from build123d import *

# Parameters (mm, degrees)
SKETCH1_W                   = 116.84
SKETCH1_H                   = 137.16
SKETCH1_R                   = 3.110430672
BOSS_EXTRUDE1_DEPTH         = 5
SKETCH12_W                  = 85
SKETCH12_H                  = 23.975046692
BOSS_EXTRUDE15_DEPTH        = 5
SKETCH17_W                  = 50
SKETCH17_H                  = 50
BOSS_EXTRUDE18_DEPTH        = 6
SKETCH10_W                  = 43
SKETCH10_H                  = 43
BOSS_EXTRUDE19_DEPTH        = 25
SKETCH19_W                  = 55
SKETCH19_H                  = 55
BOSS_EXTRUDE20_DEPTH        = 11
SKETCH20_R                  = 2.25
BOSS_EXTRUDE22_DEPTH        = 25
BOSS_EXTRUDE22_2_DEPTH      = 25
BOSS_EXTRUDE22_3_DEPTH      = 25
BOSS_EXTRUDE22_4_DEPTH      = 25
SKETCH21_W                  = 24.5
SKETCH21_H                  = 21.5
BOSS_EXTRUDE23_DEPTH        = 4
SKETCH21_W_2                = 21.5
SKETCH21_H_2                = 24.5
BOSS_EXTRUDE23_2_DEPTH      = 4
BOSS_EXTRUDE23_3_DEPTH      = 4
BOSS_EXTRUDE23_4_DEPTH      = 4
SKETCH25_R                  = 4
BOSS_EXTRUDE24_DEPTH        = 10
BOSS_EXTRUDE24_DEPTH_BACK   = 3.25
BOSS_EXTRUDE24_2_DEPTH      = 10
BOSS_EXTRUDE24_2_DEPTH_BACK = 3.25
BOSS_EXTRUDE24_3_DEPTH      = 10
BOSS_EXTRUDE24_3_DEPTH_BACK = 3.25
BOSS_EXTRUDE24_4_DEPTH      = 10
BOSS_EXTRUDE24_4_DEPTH_BACK = 3.25


with BuildPart() as part:
    # Sketch1 → Boss-Extrude1 (new body)
    with BuildSketch(Plane(origin=(0, 0, 0), x_dir=(1, 0, 0), z_dir=(0, 1, 0))):
        with Locations((-0.693486938, -16.384561015)):
            Rectangle(SKETCH1_W, SKETCH1_H)
        with Locations((-51.493486938, 44.575438985)):
            Circle(SKETCH1_R, mode=Mode.SUBTRACT)
        with Locations((50.106513062, -57.024561015)):
            Circle(SKETCH1_R, mode=Mode.SUBTRACT)
        with Locations((-51.493486938, -57.024561015)):
            Circle(SKETCH1_R, mode=Mode.SUBTRACT)
        with Locations((50.106513062, 44.575438985)):
            Circle(SKETCH1_R, mode=Mode.SUBTRACT)
    extrude(amount=-BOSS_EXTRUDE1_DEPTH)


with BuildPart() as body_2:
    # Sketch12 → Boss-Extrude15 (new body)
    with BuildSketch(Plane(origin=(0, 0, 0), x_dir=(1, 0, 0), z_dir=(0, 1, 0))):
        with Locations((0, 58)):
            Rectangle(SKETCH12_W, SKETCH12_H)
    extrude(amount=BOSS_EXTRUDE15_DEPTH)


with BuildPart() as body_3:
    # Sketch17 → Boss-Extrude18 (new body)
    with BuildSketch(Plane(origin=(0, 0, 0), x_dir=(1, 0, 0), z_dir=(0, 1, 0))):
        with Locations((-0.7, -7.31)):
            Rectangle(SKETCH17_W, SKETCH17_H)
    extrude(amount=-BOSS_EXTRUDE18_DEPTH)


with BuildPart() as body_4:
    # Sketch10 → Boss-Extrude19 (new body, symmetric)
    with BuildSketch(Plane(origin=(0, 0, 0), x_dir=(1, 0, 0), z_dir=(0, 1, 0))):
        with Locations((-0.695517903, -7.307291257)):
            Rectangle(SKETCH10_W, SKETCH10_H)
    extrude(amount=BOSS_EXTRUDE19_DEPTH, both=True)


with BuildPart() as body_5:
    # Sketch19 → Boss-Extrude20 (new body)
    with BuildSketch(Plane(origin=(0, 0, 0), x_dir=(1, 0, 0), z_dir=(0, 1, 0))):
        with Locations((-0.7, -7.31)):
            Rectangle(SKETCH19_W, SKETCH19_H)
    extrude(amount=-BOSS_EXTRUDE20_DEPTH)


with BuildPart() as part_1:
    add(part.part)

    # Combine1: cut body 2
    add(body_2.part, mode=Mode.SUBTRACT)


with BuildPart() as body_3_1:
    # Body-Move/Copy4: moved
    add(body_3.part.moved(Location((0, -6, 0))))


with BuildPart() as body_5_1:
    add(body_5.part)

    # Combine4: cut body 3
    add(body_3_1.part, mode=Mode.SUBTRACT)

    # Combine7: union part
    add(part_1.part)

    # Combine8: cut body 4
    add(body_4.part, mode=Mode.SUBTRACT)


with BuildPart() as body_2_2:
    # Sketch20 → Boss-Extrude22 (new body, symmetric)
    with BuildSketch(Plane(origin=(0, 0, 0), x_dir=(1, 0, 0), z_dir=(0, 1, 0))):
        with Locations((33.02, 33.02)):
            Circle(SKETCH20_R)
    extrude(amount=BOSS_EXTRUDE22_DEPTH, both=True)


with BuildPart() as body_3_2:
    # Sketch20 → Boss-Extrude22 2 (new body, symmetric)
    with BuildSketch(Plane(origin=(0, 0, 0), x_dir=(1, 0, 0), z_dir=(0, 1, 0))):
        with Locations((33.02, -33.02)):
            Circle(SKETCH20_R)
    extrude(amount=BOSS_EXTRUDE22_2_DEPTH, both=True)


with BuildPart() as body_4_2:
    # Sketch20 → Boss-Extrude22 3 (new body, symmetric)
    with BuildSketch(Plane(origin=(0, 0, 0), x_dir=(1, 0, 0), z_dir=(0, 1, 0))):
        with Locations((-33.02, -33.02)):
            Circle(SKETCH20_R)
    extrude(amount=BOSS_EXTRUDE22_3_DEPTH, both=True)


with BuildPart() as body_5_2:
    # Sketch20 → Boss-Extrude22 4 (new body, symmetric)
    with BuildSketch(Plane(origin=(0, 0, 0), x_dir=(1, 0, 0), z_dir=(0, 1, 0))):
        with Locations((-33.02, 33.02)):
            Circle(SKETCH20_R)
    extrude(amount=BOSS_EXTRUDE22_4_DEPTH, both=True)


with BuildPart() as body_5_3:
    add(body_5_1.part)

    # Combine9: cut body 4 2, body 3 2, body 2 2, body 5 2
    add(body_4_2.part, mode=Mode.SUBTRACT)
    add(body_3_2.part, mode=Mode.SUBTRACT)
    add(body_2_2.part, mode=Mode.SUBTRACT)
    add(body_5_2.part, mode=Mode.SUBTRACT)


with BuildPart() as body_2_3:
    # Sketch21 → Boss-Extrude23 (new body)
    with BuildSketch(Plane(origin=(0, 0, 0), x_dir=(1, 0, 0), z_dir=(0, 1, 0))):
        with Locations((-0.69, 27.145438985)):
            Rectangle(SKETCH21_W, SKETCH21_H)
    extrude(amount=-BOSS_EXTRUDE23_DEPTH)


with BuildPart() as body_3_3:
    # Sketch21 → Boss-Extrude23 2 (new body)
    with BuildSketch(Plane(origin=(0, 0, 0), x_dir=(1, 0, 0), z_dir=(0, 1, 0))):
        with Locations((32.676513062, -6.25)):
            Rectangle(SKETCH21_W_2, SKETCH21_H_2)
    extrude(amount=-BOSS_EXTRUDE23_2_DEPTH)


with BuildPart() as body_4_3:
    # Sketch21 → Boss-Extrude23 3 (new body)
    with BuildSketch(Plane(origin=(0, 0, 0), x_dir=(1, 0, 0), z_dir=(0, 1, 0))):
        with Locations((-34.063486938, -6.25)):
            Rectangle(SKETCH21_W_2, SKETCH21_H_2)
    extrude(amount=-BOSS_EXTRUDE23_3_DEPTH)


with BuildPart() as body_5_3_1:
    # Sketch21 → Boss-Extrude23 4 (new body)
    with BuildSketch(Plane(origin=(0, 0, 0), x_dir=(1, 0, 0), z_dir=(0, 1, 0))):
        with Locations((-0.69, -39.614561015)):
            Rectangle(SKETCH21_W, SKETCH21_H)
    extrude(amount=-BOSS_EXTRUDE23_4_DEPTH)


with BuildPart() as body_5_4:
    add(body_5_3.part)

    # Combine10: cut body 3 3, body 2 3, body 5 3, body 4 3
    add(body_3_3.part, mode=Mode.SUBTRACT)
    add(body_2_3.part, mode=Mode.SUBTRACT)
    add(body_5_3_1.part, mode=Mode.SUBTRACT)
    add(body_4_3.part, mode=Mode.SUBTRACT)


with BuildPart() as body_2_4:
    # Sketch25 → Boss-Extrude24 (new body, two sides)
    with BuildSketch(Plane(origin=(0, 0, 0), x_dir=(1, 0, 0), z_dir=(0, 1, 0))) as boss_extrude24_sk:
        with Locations((33.02, 33.02)):
            Circle(SKETCH25_R)
    extrude(amount=BOSS_EXTRUDE24_DEPTH)
    extrude(boss_extrude24_sk.sketch, amount=-BOSS_EXTRUDE24_DEPTH_BACK)


with BuildPart() as body_3_4:
    # Sketch25 → Boss-Extrude24 2 (new body, two sides)
    with BuildSketch(Plane(origin=(0, 0, 0), x_dir=(1, 0, 0), z_dir=(0, 1, 0))) as boss_extrude24_2_sk:
        with Locations((-33.02, 33.02)):
            Circle(SKETCH25_R)
    extrude(amount=BOSS_EXTRUDE24_2_DEPTH)
    extrude(boss_extrude24_2_sk.sketch, amount=-BOSS_EXTRUDE24_2_DEPTH_BACK)


with BuildPart() as body_4_4:
    # Sketch25 → Boss-Extrude24 3 (new body, two sides)
    with BuildSketch(Plane(origin=(0, 0, 0), x_dir=(1, 0, 0), z_dir=(0, 1, 0))) as boss_extrude24_3_sk:
        with Locations((-33.02, -33.02)):
            Circle(SKETCH25_R)
    extrude(amount=BOSS_EXTRUDE24_3_DEPTH)
    extrude(boss_extrude24_3_sk.sketch, amount=-BOSS_EXTRUDE24_3_DEPTH_BACK)


with BuildPart() as body_5_4_1:
    # Sketch25 → Boss-Extrude24 4 (new body, two sides)
    with BuildSketch(Plane(origin=(0, 0, 0), x_dir=(1, 0, 0), z_dir=(0, 1, 0))) as boss_extrude24_4_sk:
        with Locations((33.02, -33.02)):
            Circle(SKETCH25_R)
    extrude(amount=BOSS_EXTRUDE24_4_DEPTH)
    extrude(boss_extrude24_4_sk.sketch, amount=-BOSS_EXTRUDE24_4_DEPTH_BACK)


with BuildPart() as body_5_5:
    add(body_5_4.part)

    # Combine11: cut body 4 4, body 3 4, body 2 4, body 5 4
    add(body_4_4.part, mode=Mode.SUBTRACT)
    add(body_3_4.part, mode=Mode.SUBTRACT)
    add(body_2_4.part, mode=Mode.SUBTRACT)
    add(body_5_4_1.part, mode=Mode.SUBTRACT)


solid = body_5_5.part
CAD build for the part. Positions are in the model's coordinates, mm. A direction names the side the tool comes from. Coordinates: 2 decimals unless noted, no trailing zeros. Loops run counter-clockwise (first coordinate to the right, second up) from the corner with the lowest first, then second, coordinate; pieces in that order, holes last. Notation, with made-up numbers: (-33, 87.25) - (1, 87.25) arc R32 cw to (1, 113.25) - close; hole circle Ø10 at (36.5, 59). An arc over 180 degrees is marked (long way). Write item = value, one per line. Start each with the question number.
Q1. Drill centre lines: L1, parallel to Z at x = -33.02, y = -1.35; L2, parallel to Z at x = -33.02, y = -4.4; L3, parallel to X at y = -3.75, z = 33.02. Where is each one in solid material? Low to high.
Q2. Cut at B-B, the plane z = 20.5. List the corners of the cut face in (x, y), then the cut area to 3 significant figures.
Q3. Flat gauge pins, fed straight in: pin 1 Ø10 at (x, z) = (-47, 7) entering from +Y; pin 2 Ø5 at (x, z) = (33.02, 33.02) entering from -Y; pin 3 Ø2.5 at (x, y) = (-7.5, -9.5) entering from +Z; pin 4 Ø2 at (x, y) = (-34, -7.5) entering from -Z. Where does each tip first touch, or does it go through?
Q4. Pull direction Z, two halves, no side cores. Call faces 1 (the flat face through (-12.94, -2, -27)), 2 (the flat face through (-1, -8, -20.19)), 3 (the flat face through (57.727, -2, 17)): pulls with the +Z half, pulls with the -Z half, needs draft (parallel to the pull), parting line crosses it, or undercut.
Q5. Cut at D-D, the plane z = -33.02. List the corners of the cut face in (x, y), then the cut area to 3 significant figures.
Q6. Cut at C-C, the plane x = 33.02. List the corners of the cut face in (y, z), then the cut area to 3 significant figures.
Q7. Cut at A-A, the plane x = 8. List the corners of the cut face in (y, z), then the cut area to 3 significant figures.
Q8. Which spindle directions (+Z, -Z, +X, -X, +Y, -Y) get a long thin tool onto all of the face, cutting with end or side? Do faces 4 (the flat face through (-31, -3.25, -31)), 5 (the flat face through (-1, -4.3, 28.807)), 6 (the flat face through (-2, -2, 84.965)), 7 (the flat face through (-1, -8, 34.81)), 8 (the flat face through (24.3, -8, 8)). Say none if no direction does.
Computed:
q1.L1 = -52.2 to -37.02, -29.02 to -6, 18.5 to 29.02, 37.02 to 84.96
q1.L2 = -52.2 to -35.27, -30.77 to 30.77, 35.27 to 84.96
q1.L3 = -59.11 to -35.27, -30.77 to -12.94, 11.56 to 30.77, 35.27 to 57.73
q2.outline = (-59.11, -5) - (-28.2, -5) - (-28.2, -11) - (-25.7, -11) - (-25.7, -6) - (-22.2, -6) - (-22.2, 0) - (-59.11, 0) - close; (20.8, -6) - (24.3, -6) - (24.3, -11) - (26.8, -11) - (26.8, -5) - (57.73, -5) - (57.73, 0) - (20.8, 0) - close
q2.area = 406 mm²
q3.pin_1 = 0
q3.pin_2 = -5
q3.pin_3 = 34.81
q3.pin_4 = through
q4.face_1 = undercut
q4.face_2 = pulls with the -Z half
q4.face_3 = needs draft
q5.outline = (-59.11, -5) - (-35.27, -5) - (-35.27, -3.25) - (-37.02, -3.25) - (-37.02, 0) - (-59.11, 0) - close; (-30.77, -5) - (30.77, -5) - (30.77, -3.25) - (29.02, -3.25) - (29.02, 0) - (11.56, 0) - (11.56, -4) - (-12.94, -4) - (-12.94, 0) - (-29.02, 0) - (-29.02, -3.25) - (-30.77, -3.25) - close; (35.27, -5) - (57.73, -5) - (57.73, 0) - (37.02, 0) - (37.02, -3.25) - (35.27, -3.25) - close
q5.area = 418 mm²
q6.outline = (-5, -52.2) - (0, -52.2) - (0, -37.02) - (-3.25, -37.02) - (-3.25, -35.27) - (-5, -35.27) - close; (-5, -30.77) - (-3.25, -30.77) - (-3.25, -29.02) - (0, -29.02) - (0, -6) - (-4, -6) - (-4, 18.5) - (0, 18.5) - (0, 29.02) - (-3.25, 29.02) - (-3.25, 30.77) - (-5, 30.77) - close; (-5, 35.27) - (-3.25, 35.27) - (-3.25, 37.02) - (0, 37.02) - (0, 84.96) - (-5, 84.96) - close
q6.area = 520 mm²
q7.outline = (-11, -20.19) - (-5, -20.19) - (-5, -52.2) - (0, -52.2) - (0, -37.9) - (-4, -37.9) - (-4, -16.4) - (0, -16.4) - (0, -14.19) - (-6, -14.19) - (-6, -17.69) - (-11, -17.69) - close; (-11, 32.31) - (-6, 32.31) - (-6, 28.81) - (0, 28.81) - (0, 28.86) - (-4, 28.86) - (-4, 50.36) - (0, 50.36) - (0, 84.96) - (-5, 84.96) - (-5, 34.81) - (-11, 34.81) - close
q7.area = 336 mm²
q8.face_4 = +Y
q8.face_5 = +Y, -Y
q8.face_6 = +Z, +X, -X, +Y, -Y
q8.face_7 = +Z, +X, -X, -Y
q8.face_8 = -Y
